Work out the finished part from the listing and answer in its coordinate system (mm). Coordinates: 2 decimals unless noted, no trailing zeros. Write each loop counter-clockwise with the first axis right and the second up, starting at its lowest first coordinate (ties: lowest second). Pieces come first, ordered by that corner, then holes. Notation, with made-up numbers: (-22.5, 5) - (-11.5, 5) arc R24 ccw to (-11.5, 21) - close; hole circle Ø2 at (32, -39). An arc over 180 degrees is marked (long way). Use one line per item in the form item = value. Start each with the question number.
Item 1: A cutting plane is placed at D-D (z = 1.15). Give the number of separate pieces and of enclosed holes in the cut face, then the cut area to 3 significant figures.
Item 2: Determine the mould class of faces 1 (the cylindrical face through (72, 13.5, 1)), 2 (the flat face through (1, 50, 2)) for opening direction X: released by +X, released by -X, zero draft, split by the parting line, or undercut.
Item 3: A cutting plane is placed at A-A (x = -70). Write down the section's boundary in (y, z).
Item 4: A cutting plane is placed at B-B (y = 0). Write down the section's boundary in (x, z), then the cut area to 3 significant figures.
Item 5: Consider probe 1 along Y at (x, z) = (-70, 1.5); probe 2 along Y at (x, z) = (-40, 1.3); probe 3 along X at (y, z) = (-24, 1.35). Determine where each line is inside the solid, lowest interval first.
Item 6: A cutting plane is placed at C-C (x = -27). Write down the section's boundary in (y, z), then the cut area to 3 significant figures.
from build123d import *

# Parameters (mm, degrees)
PAD_DEPTH       = 2
SKETCH001_W     = 120
SKETCH001_H     = 75
POCKET_DEPTH    = 7
SKETCH002_R     = 2.5
POCKET001_DEPTH = 7
SKETCH003_R     = 2.5
POCKET002_DEPTH = 7


with BuildPart() as part:
    # Sketch → Pad (new body)
    with BuildSketch(Plane.XY):
        with BuildLine():
            Line((-97.5, 74), (97.5, 74))
            ThreePointArc((99.5, 72), (98.914214, 73.414214), (97.5, 74))
            Line((99.5, 72), (99.5, -72))
            ThreePointArc((97.5, -74), (98.914214, -73.414214), (99.5, -72))
            Line((97.5, -74), (-97.5, -74))
            ThreePointArc((-99.5, -72), (-98.914214, -73.414214), (-97.5, -74))
            Line((-99.5, -72), (-99.5, 72))
            ThreePointArc((-97.5, 74), (-98.914214, 73.414214), (-99.5, 72))
        make_face()
    extrude(amount=PAD_DEPTH)

    # Sketch001 → Pocket (cut)
    with BuildSketch(Plane.XY):
        Rectangle(SKETCH001_W, SKETCH001_H)
    extrude(amount=POCKET_DEPTH, mode=Mode.SUBTRACT)

    # Sketch002 → Pocket001 (cut)
    with BuildSketch(Plane.XY):
        with Locations((0, 47.5)):
            Circle(SKETCH002_R)
        with Locations((-40, 47.5)):
            Circle(SKETCH002_R)
        with Locations((-20, 47.5)):
            Circle(SKETCH002_R)
        with Locations((20, 47.5)):
            Circle(SKETCH002_R)
        with Locations((40, 47.5)):
            Circle(SKETCH002_R)
    extrude(amount=POCKET001_DEPTH, mode=Mode.SUBTRACT)

    # Sketch003 → Pocket002 (cut)
    with BuildSketch(Plane.XY):
        with Locations((-70, 0)):
            Circle(SKETCH003_R)
        with Locations((-70, 15)):
            Circle(SKETCH003_R)
        with Locations((-70, 30)):
            Circle(SKETCH003_R)
        with Locations((-70, -15)):
            Circle(SKETCH003_R)
        with Locations((-70, -30)):
            Circle(SKETCH003_R)
    pocket002 = extrude(amount=POCKET002_DEPTH, mode=Mode.SUBTRACT)

    # Mirrored: Pocket002 across Sketch003 V_Axis
    add(pocket002.mirror(Plane(origin=(0, 0, 0), x_dir=(0, 0, 1), z_dir=(1, 0, 0))), mode=Mode.SUBTRACT)


solid = part.part
Answer:
q1.separate_pieces = 1
q1.enclosed_holes = 16
q1.area = 20,200 mm²
q2.face_1 = undercut
q2.face_2 = zero draft
q3.outline = (-74, 0) - (-32.5, 0) - (-32.5, 2) - (-74, 2) - close; (-27.5, 0) - (-17.5, 0) - (-17.5, 2) - (-27.5, 2) - close; (-12.5, 0) - (-2.5, 0) - (-2.5, 2) - (-12.5, 2) - close; (2.5, 0) - (12.5, 0) - (12.5, 2) - (2.5, 2) - close; (17.5, 0) - (27.5, 0) - (27.5, 2) - (17.5, 2) - close; (32.5, 0) - (74, 0) - (74, 2) - (32.5, 2) - close
q4.outline = (-99.5, 0) - (-72.5, 0) - (-72.5, 2) - (-99.5, 2) - close; (-67.5, 0) - (-60, 0) - (-60, 2) - (-67.5, 2) - close; (60, 0) - (67.5, 0) - (67.5, 2) - (60, 2) - close; (72.5, 0) - (99.5, 0) - (99.5, 2) - (72.5, 2) - close
q4.area = 138 mm²
q5.probe_1 = -74 to -32.5, -27.5 to -17.5, -12.5 to -2.5, 2.5 to 12.5, 17.5 to 27.5, 32.5 to 74
q5.probe_2 = -74 to -37.5, 37.5 to 45, 50 to 74
q5.probe_3 = -99.5 to -60, 60 to 99.5
q6.outline = (-74, 0) - (-37.5, 0) - (-37.5, 2) - (-74, 2) - close; (37.5, 0) - (74, 0) - (74, 2) - (37.5, 2) - close
q6.area = 146 mm²
